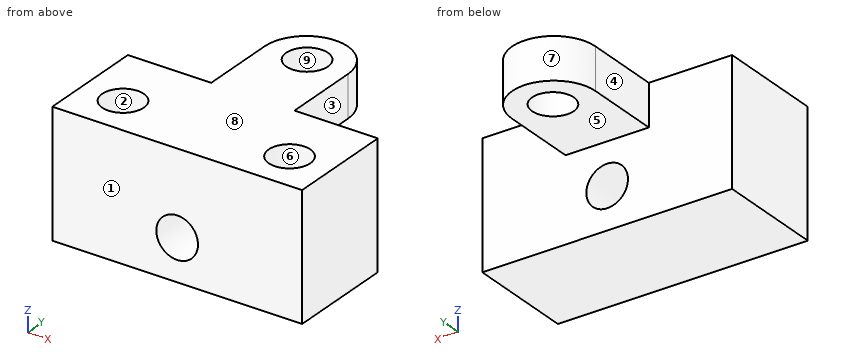
from build123d import *

# Parameters (mm, degrees)
F0_W      = 160
F0_H      = 160
F1_DEPTH  = 160
F4_W      = 300
F4_H      = 150
F5_DEPTH  = 130
F6_W      = 100
F6_H      = 143
F7_DEPTH  = 50
F8_R      = 25
F9_DEPTH  = 100
F10_R     = 25
F11_DEPTH = 50
F13_DEPTH = 50
F14_R     = 25
F15_DEPTH = 130


with BuildPart() as f1:
    # F0 (on Front) → F1 (new body)
    with BuildSketch(Plane.XZ):
        Rectangle(F0_W, F0_H)
    extrude(amount=F1_DEPTH)


with BuildPart() as f5:
    # F4 (on face) → F5 (new body)
    with BuildSketch(Plane(origin=(0, 0, 0), x_dir=(-1, 0, 0), z_dir=(0, 1, 0))):
        Rectangle(F4_W, F4_H)
    extrude(amount=F5_DEPTH)

    # F6 (on face) → F7 (join)
    with BuildSketch(Plane.XY.offset(75)):
        with Locations((0, 201.5)):
            Rectangle(F6_W, F6_H)
    extrude(amount=-F7_DEPTH)

    # F8 (on face) → F9 (cut)
    with BuildSketch(Plane.XY.offset(75)):
        with Locations((100, 50)):
            Circle(F8_R)
        with Locations((-100, 50)):
            Circle(F8_R)
    extrude(amount=-F9_DEPTH, mode=Mode.SUBTRACT)

    # F10 (on face) → F11 (cut)
    with BuildSketch(Plane.XY.offset(75)):
        with Locations((0, 223.2050807569)):
            Circle(F10_R)
    extrude(amount=-F11_DEPTH, mode=Mode.SUBTRACT)

    # F12 (on face) → F13 (cut)
    with BuildSketch(Plane.XY.offset(75)):
        with BuildLine():
            ThreePointArc((-50, 221.6448485851), (0, 271.6448485851), (50, 221.6448485851))
            Line((50, 221.6448485851), (50, 273))
            Line((50, 273), (-50, 273))
            Line((-50, 273), (-50, 221.6448485851))
        make_face()
    extrude(amount=-F13_DEPTH, mode=Mode.SUBTRACT)

    # F14 (on face) → F15 (cut)
    with BuildSketch(Plane.XZ):
        with Locations((0, -25)):
            Circle(F14_R)
    extrude(amount=-F15_DEPTH, mode=Mode.SUBTRACT)


solid = f5.part
Geometry check sheet. Reference: the model listing, model coordinates, mm. Face numbers are marked on the shaded views. A direction names the side the tool comes from. Give positions to 0.01 mm unless a question says otherwise; leave off trailing zeros. Loops run counter-clockwise (first coordinate to the right, second up) from the corner with the lowest first, then second, coordinate; pieces in that order, holes last. Notation, with made-up numbers: (87, -24) -> (92, -24) arc R28 cw to (92, 15) -> close; hole circle Ø6 at (13.5, 52). An arc over 180 degrees is marked (long way). Answer in a Markdown table with one row per item. Add a question column.
1) Cross-section at A-A on x = 0. Record the boundary of the cut face in (y, z), and give its area (3 significant figures).
2) Material ranges on probe 1 along Z at (x, y) = (5.5, 159); probe 2 along Y at (x, z) = (-111.5, -59.5); probe 3 along Y at (x, z) = (0, 35.5), recorded low to high. Write a range as from..to.
3) Cross-section at D-D on x = 100. Record the boundary of the cut face in (y, z), and give its area (3 significant figures).
4) Gauge pin test, flat ends, axial feed: P1, Ø3, axis at x = 74, z = -4.5, coming from the +Y side; P2, Ø15, axis at y = 157, z = 50.5, coming from the -X side; P3, Ø15, axis at x = 88, y = 47.5, coming from the +Z side. Record the tip position at first contact, or that the pin passes through.
5) Draft check along Y on the marked faces 6, 7, 8 and 9. Enter one of: pulls with the +Y half, pulls with the -Y half, needs draft (parallel to the pull), parting line crosses it, or undercut.
6) Set-up check for the marked faces 1, 2, 3, 4 and 5: record each of +Z, -Z, +X, -X, +Y, -Y from which the full face is reachable in a straight line by a thin tool's end or side.
7) Cross-section at B-B on y = 50. Record the boundary of the cut face in (x, z), and give its area (3 significant figures).
8) Cross-section at C-C on y = 218. Record the boundary of the cut face in (x, z), and give its area (3 significant figures).
Outcome:
| question | item | result |
|---|---|---|
| 1 | outline | (0, -75) -> (130, -75) -> (130, -50) -> (0, -50) -> close; (0, 0) -> (130, 0) -> (130, 25) -> (198.21, 25) -> (198.21, 75) -> (0, 75) -> close; (248.21, 25) -> (271.64, 25) -> (271.64, 75) -> (248.21, 75) -> close |
| 1 | area | 17,600 mm^2 |
| 2 | probe 1 | z = 25..75 |
| 2 | probe 2 | y = 0..130 |
| 2 | probe 3 | y = 0..198.21, 248.21..271.64 |
| 3 | outline | (0, -75) -> (130, -75) -> (130, 75) -> (75, 75) -> (75, -25) -> (25, -25) -> (25, 75) -> (0, 75) -> close |
| 3 | area | 14,500 mm^2 |
| 4 | P1 | stops at y = 130 |
| 4 | P2 | stops at x = -50 |
| 4 | P3 | stops at z = -25 |
| 5 | face 6 | undercut |
| 5 | face 7 | pulls with the +Y half |
| 5 | face 8 | needs draft |
| 5 | face 9 | undercut |
| 6 | face 1 | +Z, -Z, +X, -X, -Y |
| 6 | face 2 | +Z |
| 6 | face 3 | +Z, -Z, +X, +Y |
| 6 | face 4 | +Z, -Z, -X, +Y |
| 6 | face 5 | -Z, +X, -X, +Y |
| 7 | outline | (-150, -75) -> (150, -75) -> (150, 75) -> (125, 75) -> (125, -25) -> (75, -25) -> (75, 75) -> (-75, 75) -> (-75, -25) -> (-125, -25) -> (-125, 75) -> (-150, 75) -> close; hole circle Ø50 at (0, -25) |
| 7 | area | 33,000 mm^2 |
| 8 | outline | (-50, 25) -> (-24.45, 25) -> (-24.45, 75) -> (-50, 75) -> close; (24.45, 25) -> (50, 25) -> (50, 75) -> (24.45, 75) -> close |
| 8 | area | 2,550 mm^2 |
